```python
from build123d import *

# Parameters (mm, degrees)
BOSS_EXTRUDE1_DEPTH     = 20
SKETCH2_R               = 2
CUT_EXTRUDE1_DEPTH      = 20
SKETCH3_R               = 3
CUT_EXTRUDE2_DEPTH      = 13.5
SKETCH4_OUTSIDE_W       = 74.532
SKETCH4_OUTSIDE_H       = 76.178
SKETCH4_OUTSIDE_R       = 5.878507538
CUT_EXTRUDE3_DEPTH      = 23.027138831
CUT_EXTRUDE3_DRAFT      = -50
MIRROR1_COPY_1_SKETCH_W = 74.532
MIRROR1_COPY_1_SKETCH_H = 76.178
MIRROR1_COPY_1_SKETCH_R = 5.878507538
MIRROR1_COPY_1_DEPTH    = 23.027138831
MIRROR1_COPY_1_DRAFT    = -50
CUT_EXTRUDE4_REACH      = 27.108
CUT_EXTRUDE4_END_RADIUS = 3
SKETCH5_R               = 1.25


with BuildPart() as part:
    # Sketch1 → Boss-Extrude1 (new body)
    with BuildSketch(Plane.XY):
        Polygon((-6.102382196, -3.280385881), (-0.210293591, -6.925010946), (5.892088606, -3.644625065), (6.102382196, 3.280385881), (0.210293591, 6.925010946), (-5.892088606, 3.644625065), align=None)
    extrude(amount=BOSS_EXTRUDE1_DEPTH)

    # Sketch2 → Cut-Extrude1 (cut)
    with BuildSketch(Plane(origin=(0, 0, 0), x_dir=(-1, 0, 0), z_dir=(0, 0, -1))):
        Circle(SKETCH2_R)
    extrude(amount=-CUT_EXTRUDE1_DEPTH, mode=Mode.SUBTRACT)

    # Sketch3 → Cut-Extrude2 (cut)
    with BuildSketch(Plane.XY.offset(20)):
        Circle(SKETCH3_R)
    extrude(amount=-CUT_EXTRUDE2_DEPTH, mode=Mode.SUBTRACT)


with BuildPart() as cut_extrude3_tool:
    # Sketch4 outside → Cut-Extrude3 (with draft: the straight prism first)
    with BuildSketch(Plane.XY.offset(20)):
        Rectangle(SKETCH4_OUTSIDE_W, SKETCH4_OUTSIDE_H)
        Circle(SKETCH4_OUTSIDE_R, mode=Mode.SUBTRACT)
    extrude(amount=-CUT_EXTRUDE3_DEPTH)
    # Cut-Extrude3: the draft: its side faces are tilted about the plane it starts from
    cut_extrude3_sides = [cut_extrude3_tool.faces().sort_by_distance(p)[0] for p in [
        (0, -38.089, 8.486430585),
        (37.266, 0, 8.486430585),
        (0, 38.089, 8.486430585),
        (-37.266, 0, 8.486430585),
        (-5.878507538, 0, 8.486430585),
    ]]
    draft(cut_extrude3_sides, Plane.XY.offset(20), CUT_EXTRUDE3_DRAFT)


with BuildPart() as part_1:
    add(part.part)

    # Cut-Extrude3: cut by cut_extrude3_tool
    add(cut_extrude3_tool.part, mode=Mode.SUBTRACT)


with BuildPart() as mirror1_copy_1_tool:
    # Mirror1 copy 1 sketch → Mirror1 copy 1 (with draft: the straight prism first)
    with BuildSketch(Plane(origin=(0, 0, 0), x_dir=(1, 0, 0), z_dir=(0, 0, -1))):
        Rectangle(MIRROR1_COPY_1_SKETCH_W, MIRROR1_COPY_1_SKETCH_H)
        Circle(MIRROR1_COPY_1_SKETCH_R, mode=Mode.SUBTRACT)
    extrude(amount=-MIRROR1_COPY_1_DEPTH)
    # Mirror1 copy 1: the draft: its side faces are tilted about the plane it starts from
    mirror1_copy_1_sides = [mirror1_copy_1_tool.faces().sort_by_distance(p)[0] for p in [
        (0, -38.089, 11.513569415),
        (37.266, 0, 11.513569415),
        (0, 38.089, 11.513569415),
        (-37.266, 0, 11.513569415),
        (-5.878507538, 0, 11.513569415),
    ]]
    draft(mirror1_copy_1_sides, Plane(origin=(0, 0, 0), x_dir=(1, 0, 0), z_dir=(0, 0, -1)), MIRROR1_COPY_1_DRAFT)


with BuildPart() as part_2:
    add(part_1.part)

    # Mirror1 copy 1: cut by mirror1_copy_1_tool
    add(mirror1_copy_1_tool.part, mode=Mode.SUBTRACT)

    # Cut-Extrude4: up to this cylinder (the profile starts outside it)
    cut_extrude4_end = Plane(origin=(0, 0, 15), z_dir=(0, 0, 1)) * Cylinder(CUT_EXTRUDE4_END_RADIUS, 65.216, mode=Mode.PRIVATE)
    # Sketch5 → Cut-Extrude4 (cut, up to the surface)
    with BuildSketch(Plane(origin=(3.156337894, 5.102698414, 0), x_dir=(0.8504497356266733, -0.5260563155903765, 0), z_dir=(0.5260563155903764, 0.8504497356266731, 0)), mode=Mode.PRIVATE) as cut_extrude4_sk1:
        with Locations(Location((0, -17, 0), (0, 0, 180))):
            Circle(SKETCH5_R)
    cut_extrude4_tool1 = extrude(cut_extrude4_sk1.sketch, amount=-CUT_EXTRUDE4_REACH, mode=Mode.PRIVATE) - cut_extrude4_end
    add(cut_extrude4_tool1.solids().sort_by_distance((3.156338, 5.102698, 17))[0], mode=Mode.SUBTRACT)
    # Sketch5 → Cut-Extrude4 (cut, up to the surface)
    with BuildSketch(Plane(origin=(3.156337894, 5.102698414, 0), x_dir=(0.8504497356266733, -0.5260563155903765, 0), z_dir=(0.5260563155903764, 0.8504497356266731, 0)), mode=Mode.PRIVATE) as cut_extrude4_sk2:
        with Locations(Location((0, -13, 0), (0, 0, 180))):
            Circle(SKETCH5_R)
    cut_extrude4_tool2 = extrude(cut_extrude4_sk2.sketch, amount=-CUT_EXTRUDE4_REACH, mode=Mode.PRIVATE) - cut_extrude4_end
    add(cut_extrude4_tool2.solids().sort_by_distance((3.156338, 5.102698, 13))[0], mode=Mode.SUBTRACT)


solid = part_2.part
```
Work out the finished part from the listing and answer in its coordinate system (mm). A direction names the side the tool comes from. Coordinates: 2 decimals unless noted, no trailing zeros. Loops run counter-clockwise (first coordinate to the right, second up) from the corner with the lowest first, then second, coordinate; pieces in that order, holes last.
1) Section C-C (z = 13.5) is taken. Give the vertices of the cut face in (x, y), plus the area to 3 significant figures.
Results:
outline: (-6.1, -3.28) - (-0.21, -6.93) - (5.89, -3.64) - (6.1, 3.28) - (4.13, 4.5) - (2.43, 1.76) arc R3 cw (long way) to (0.48, 2.96) - (2.18, 5.71) - (0.21, 6.93) - (-5.89, 3.64) - close
area: 89.4 mm2
2) Section B-B (y = 0) is taken. Give the vertices of the cut face in (x, z), plus the area to 3 significant figures.
Results:
outline: (-6, 0.1) - (-5.88, 0) - (-2, 0) - (-2, 6.5) - (-3, 6.5) - (-3, 20) - (-5.88, 20) - (-6, 19.9) - close; (2, 0) - (5.88, 0) - (6, 0.1) - (6, 19.9) - (5.88, 20) - (3, 20) - (3, 6.5) - (2, 6.5) - close
area: 133 mm2
3) For a pull along X with two mould halves and no side action, classify faces 1 (the flat face through (-2.798, 5.308, 9.861)), 2 (the cylindrical face through (2.45, 3.64, 18.24)), 3 (the flat face through (2.798, -5.308, 9.861)) as +X half, -X half, draft (parallel to the pull), parting line (faces both ways), or undercut.
Results:
face 1: -X half
face 2: undercut
face 3: +X half
4) Section A-A (z = 4.25) is taken. Give the vertices of the cut face in (x, y), plus the area to 3 significant figures.
Results:
outline: (-6.1, -3.28) - (-0.21, -6.93) - (5.89, -3.64) - (6.1, 3.28) - (0.21, 6.93) - (-5.89, 3.64) - close; hole circle Ø4 at (0, 0)
area: 112 mm2
5) Flat-ended cylindrical pins translate along their axes: pin 1 (5 mm diameter, centred on x = 0, y = 0, fed in from +Z); pin 2 (3 mm diameter, centred on y = 2.5, z = 11.5, fed in from -X); pin 3 (3 mm diameter, centred on y = 3, z = 8, fed in from +X); pin 4 (3.5 mm diameter, centred on x = 0, y = 0, fed in from -Z). Find the tip coordinate at first contact, or state that the pin passes through.
Results:
pin 1: stops at z = 6.5
pin 2: stops at x = -5.97
pin 3: stops at x = 6.1
pin 4: passes through
6) Consider probe 1 along Y at (x, z) = (1.25, 10.5); probe 2 along Y at (x, z) = (0, 10); probe 3 along Z at (x, y) = (3, 3.5). Determine where each line is inside the solid, lowest interval first.
Results:
probe 1: y = -6.14 to -2.73, 2.73 to 6.28
probe 2: y = -6.81 to -3, 3 to 6.81
probe 3: z = 0 to 11.97, 14.03 to 15.97, 18.03 to 20
7) For faces 4 (the flat face through (-1, 3, 20)), 5 (the cylindrical face through (-2.4, -1.8, 13.3)), determine the directions among +Z, -Z, +X, -X, +Y, -Y from which every point of the face is accessible in a straight line to the end or side of a thin tool.
Results:
face 4: +Z, +X, -X, +Y, -Y
face 5: +Z
